```python
from build123d import *

# Parameters (mm, degrees)
BOSS_EXTRUDE1_DEPTH = 241
CUT_EXTRUDE1_DEPTH  = 78


with BuildPart() as part:
    # Sketch2 → Boss-Extrude1 (new body)
    with BuildSketch(Plane.XY):
        with BuildLine():
            Line((0, -28.575), (0, -82))
            Line((0, -82), (-13, -82))
            Line((-13, -82), (-82, -42.162831426))
            Line((-82, -42.162831426), (-82, 0))
            ThreePointArc((-82, 0), (-57.982756057, 57.982756057), (0, 82))
            Line((0, 82), (0, 28.575))
            ThreePointArc((0, 28.575), (-28.575, 0), (0, -28.575))
        make_face()
    extrude(amount=-BOSS_EXTRUDE1_DEPTH)

    # Sketch3 → Cut-Extrude1 (cut)
    with BuildSketch(Plane.XY):
        with BuildLine():
            Line((0, 44.45), (0, 28.575))
            ThreePointArc((0, 28.575), (-28.575, 0), (0, -28.575))
            Line((0, -28.575), (0, -44.45))
            ThreePointArc((0, -44.45), (-44.45, 0), (0, 44.45))
        make_face()
    extrude(amount=-CUT_EXTRUDE1_DEPTH, mode=Mode.SUBTRACT)


solid = part.part
```
The model under review builds one solid part; all positions refer to its coordinate system, in mm. A direction names the side the tool comes from. Round coordinates to 2 decimals unless told otherwise and drop trailing zeros. Order: outer loops, then holes, each group sorted by start corner. A loop starts at its lowest first (then second) coordinate and runs counter-clockwise, first axis right, second up. Notation, with made-up numbers: (16.5, -30) - (63.5, -30) arc R36 ccw to (63.5, 9) - close; hole circle Ø10 at (-6, -23). An arc over 180 degrees is marked (long way). Answer in a Markdown table with one row per item.
(1) Take a section at A-A on z = -201. Write out the cut boundary in (x, y) (3 decimals).
Result set:
| item | result |
|---|---|
| outline | (-82, -42.163) - (-13, -82) - (0, -82) - (0, -28.575) arc R28.575 cw to (0, 28.575) - (0, 82) arc R82 ccw to (-82, 0) - close |
(2) Take a section at D-D on y = -50. Write out the cut boundary in (x, z).
Result set:
| item | result |
|---|---|
| outline | (-68.43, -241) - (0, -241) - (0, 0) - (-68.43, 0) - close |
(3) Clearance check with flat-ended pins moving along their axes: P1, Ø10, axis at x = -50.5, z = -67, coming from the +Y side; P2, Ø6, axis at y = 10.5, z = -197, coming from the +X side; P3, Ø4, axis at y = -59.5, z = -113.5, coming from the -X side. State where each tip first meets the part, or that it passes through.
Result set:
| item | result |
|---|---|
| P1 | stops at y = 68.22 |
| P2 | stops at x = -25.18 |
| P3 | stops at x = -55.44 |
(4) Mouldability with a two-part tool opening along Y and no side actions: class faces 3 (the face through (-6, -82, -119)), 4 (the face through (-50, 1, 0)), 5 (the face through (-44.44, -0.98, -38.45)) as released by +Y, released by -Y, zero draft, split by the parting line, or undercut.
Result set:
| item | result |
|---|---|
| face 3 | released by -Y |
| face 4 | zero draft |
| face 5 | undercut |
(5) Take a section at C-C on z = -16.5. Write out the cut boundary in (x, y).
Result set:
| item | result |
|---|---|
| outline | (-82, -42.16) - (-13, -82) - (0, -82) - (0, -44.45) arc R44.45 cw to (0, 44.45) - (0, 82) arc R82 ccw to (-82, 0) - close |
(6) Take a section at B-B on x = -42. Write out the cut boundary in (y, z), plus the area to 3 significant figures.
Result set:
| item | result |
|---|---|
| outline | (-65.26, -241) - (70.43, -241) - (70.43, 0) - (14.55, 0) - (14.55, -78) - (-14.55, -78) - (-14.55, 0) - (-65.26, 0) - close |
| area | 30,400 mm2 |
(7) Machinability: for faces 1 (the face through (-58.62, 57.34, -118.81)), 2 (the face through (-32, 1, -78)), which of the approach directions +Z, -Z, +X, -X, +Y, -Y give a long, thin tool a straight path to every point of the face, cutting with its end or side? Answer none if there is none.
Result set:
| item | result |
|---|---|
| face 1 | +Z, -Z, -X, +Y |
| face 2 | +Z, +X |
(8) For line 1 (Z direction, x = -32.5, y = 28.5); line 2 (Y direction, x = -5.5, z = -80.5); line 3 (Y direction, x = -22, z = -152), list the stretches that pass through material, from the lowest coordinate up. Write a range as from..to.
Result set:
| item | result |
|---|---|
| line 1 | z = -241..-78 |
| line 2 | y = -82..-28.04, 28.04..81.82 |
| line 3 | y = -76.8..-18.24, 18.24..78.99 |
